Verification items for this drawing (mm, ordinates from the low corner). A direction names the side the tool comes from. Round coordinates to 2 decimals unless told otherwise and drop trailing zeros. Loops run counter-clockwise (first coordinate to the right, second up) from the corner with the lowest first, then second, coordinate; pieces in that order, holes last. Notation, with made-up numbers: M -30,25 L 14,25 A25 ccw 14,50 Z; hole C -12.5,41 d8. An arc over 180 degrees is marked long. Use one line per item in the form item = value. Start each with the question number.
1. Material ranges on line 1 (X direction, y = 6, z = 3.5); line 2 (Y direction, x = 51.6, z = 17.4); line 3 (X direction, y = 2.25, z = 10), recorded low to high.
2. Cross-section at C-C (x = 20.6). Record the boundary of the cut face in (y, z).
3. Go/stop test with flat-tipped pins: pin 1 (4 mm diameter, centred on x = 8.5, y = 10, fed in from +Z); pin 2 (6.5 mm diameter, centred on x = 51.6, y = 6, fed in from -Z); pin 3 (4.5 mm diameter, centred on x = 5, y = 6, fed in from +Z); pin 4 (6.5 mm diameter, centred on x = 66, y = 5.5, fed in from +Z). Record where each tip stops, or that it passes through.
4. Cross-section at D-D (y = 6). State how many separate pieces and enclosed holes the cut face has, then the cut area to 3 significant figures.
5. Cross-section at B-B (y = 1). Record the boundary of the cut face in (x, z).
6. Set-up check for the marked faces 1, 2 and 3: record each of +Z, -Z, +X, -X, +Y, -Y from which the full face is reachable in a straight line by a thin tool's end or side.
7. Cross-section at A-A (z = 13.25). Record the boundary of the cut face in (x, y).
8. Draft check along X on the marked faces 4, 5 and 6. Enter one of: pulls with the +X half, pulls with the -X half, needs draft (parallel to the pull), parting line crosses it, or undercut.
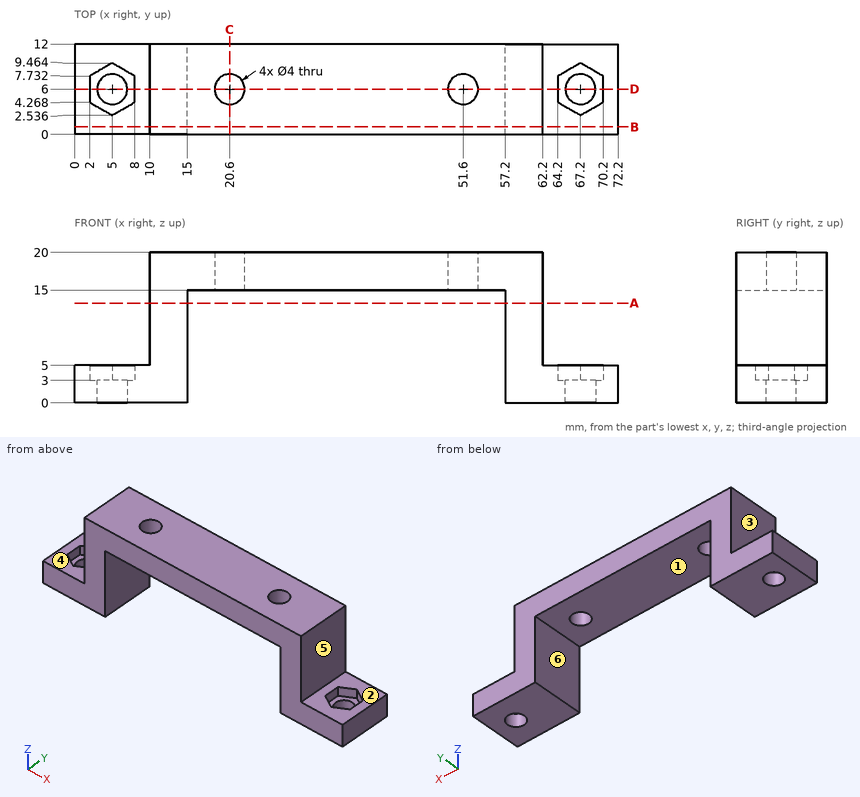
Reported:
q1.line_1 = 0 to 2, 8 to 15, 57.2 to 64.2, 70.2 to 72.2
q1.line_2 = 0 to 4, 8 to 12
q1.line_3 = 10 to 15, 57.2 to 62.2
q2.outline = M 0,15 L 4,15 L 4,20 L 0,20 Z; M 8,15 L 12,15 L 12,20 L 8,20 Z
q3.pin_1 = 20
q3.pin_2 = 15
q3.pin_3 = 3
q3.pin_4 = 5
q4.separate_pieces = 5
q4.enclosed_holes = 0
q4.area = 423 mm²
q5.outline = M 0,0 L 15,0 L 15,15 L 57.2,15 L 57.2,0 L 72.2,0 L 72.2,5 L 62.2,5 L 62.2,20 L 10,20 L 10,5 L 0,5 Z
q6.face_1 = -Z, +Y, -Y
q6.face_2 = +Z, +X, +Y, -Y
q6.face_3 = +Z, -X, +Y, -Y
q7.outline = M 10,0 L 15,0 L 15,12 L 10,12 Z; M 57.2,0 L 62.2,0 L 62.2,12 L 57.2,12 Z
q8.face_4 = needs draft
q8.face_5 = pulls with the +X half
q8.face_6 = undercut
